```python
from build123d import *

# Parameters (mm, degrees)
SKETCH1_R                          = 76.2
MAIN_EXTRUDE_DEPTH                 = 50.5582
SKETCH4_R                          = 76.2
SKETCH4_R_2                        = 75.057
TURN_OUTSIDE_DEPTH                 = 37.846
SKETCH5_R                          = 74.295
EXTRUDE1_DEPTH                     = 0.9906
SKETCH7_R                          = 76.2
FACE_BOTTOM_DEPTH                  = 1.5367
SKETCH8_R                          = 76.2
SKETCH8_R_2                        = 75.057
TURN_REST_OF_OUTSIDE_DEPTH         = 12.1755
SKETCH3_R                          = 2.3876
PILOT_HOLE_FOR_BALL_DEPTH          = 12.446
SPHERICAL_BALL_ANGLE               = 180
CHAMFER1_SIZE                      = 16.002
F_5_16_0_3125_DIAMETER_HOLE1_D     = 7.9375
F_5_16_0_3125_DIAMETER_HOLE1_DEPTH = 0.508
RETAINER_HOLE_PATTERN_COUNT        = 3
M5X0_8_TAPPED_HOLE1_D              = 4.2
M5X0_8_TAPPED_HOLE1_DEPTH          = 66.675
M5X0_8_TAPPED_HOLE1_TIP            = 1.2618073


with BuildPart() as part:
    # Sketch1 → Main Extrude (new body)
    with BuildSketch(Plane(origin=(0, 0, 0), x_dir=(1, 0, 0), z_dir=(0, 1, 0))):
        with Locations(Location((0, 0, 0), (0, 0, 270))):  # turned: the seam where the file's is
            Circle(SKETCH1_R)
    extrude(amount=MAIN_EXTRUDE_DEPTH)

    # Sketch4 → Turn Outside (cut)
    with BuildSketch(Plane.XZ):
        with Locations(Location((0, 0, 0), (0, 0, 270))):  # turned: the seam where the file's is
            Circle(SKETCH4_R)
        with Locations(Location((0, 0, 0), (0, 0, 270))):  # turned: the seam where the file's is
            Circle(SKETCH4_R_2, mode=Mode.SUBTRACT)
    extrude(amount=-TURN_OUTSIDE_DEPTH, mode=Mode.SUBTRACT)

    # Sketch5 → Extrude1 (add)
    with BuildSketch(Plane.XZ):
        with Locations(Location((0, 0, 0), (0, 0, 90))):  # turned: the seam where the file's is
            Circle(SKETCH5_R)
    extrude(amount=EXTRUDE1_DEPTH)

    # Sketch7 → Face Bottom (cut)
    with BuildSketch(Plane(origin=(0, 50.5582, 0), x_dir=(-1, 0, 0), z_dir=(0, 1, 0))):
        with Locations(Location((0, 0, 0), (0, 0, 270))):  # turned: the seam where the file's is
            Circle(SKETCH7_R)
    extrude(amount=-FACE_BOTTOM_DEPTH, mode=Mode.SUBTRACT)

    # Sketch8 → Turn rest of outside (cut, through all)
    with BuildSketch(Plane.XZ.offset(-37.846)):
        Circle(SKETCH8_R)
        with Locations(Location((0, 0, 0), (0, 0, 270))):  # turned: the seam where the file's is
            Circle(SKETCH8_R_2, mode=Mode.SUBTRACT)
    extrude(amount=-TURN_REST_OF_OUTSIDE_DEPTH, mode=Mode.SUBTRACT)

    # Sketch3 → Pilot hole for ball (cut)
    with BuildSketch(Plane(origin=(0, 49.0215, 0), x_dir=(-1, 0, 0), z_dir=(0, 1, 0))):
        with Locations(Location((0, 0, 0), (0, 0, 90))):  # turned: the seam where the file's is
            Circle(SKETCH3_R)
    extrude(amount=-PILOT_HOLE_FOR_BALL_DEPTH, mode=Mode.SUBTRACT)

    # Sketch2 → Spherical Ball (revolve, cut)
    with BuildSketch(Plane(origin=(0, 49.5295, 0), x_dir=(-1, 0, 0), z_dir=(0, 1, 0))):
        with BuildLine():
            Line((12.499975, 0), (-12.499975, 0))
            ThreePointArc((-12.499975, 0), (0, -12.499975), (12.499975, 0))
        make_face()
    revolve(axis=Axis((-12.499975, 49.5295, 0), (-1, 0, 0)), revolution_arc=SPHERICAL_BALL_ANGLE, mode=Mode.SUBTRACT)

    # Chamfer1
    chamfer1_edges = [part.edges().sort_by_distance(p)[0] for p in [
        (0, 49.0215, 75.057),
    ]]
    chamfer(chamfer1_edges, length=CHAMFER1_SIZE)

    # 5_16 _0.3125_ Diameter Hole1
    with Locations(Plane(origin=(75.184, 0, 0), x_dir=(0, 0, -1), z_dir=(1, 0, 0))):
        with Locations((0, 7.5179)):
            Hole(F_5_16_0_3125_DIAMETER_HOLE1_D / 2, depth=F_5_16_0_3125_DIAMETER_HOLE1_DEPTH)

    # Sketch15 → M3x0.5 Retainer Hole (revolve, cut)
    with BuildSketch(Plane(origin=(-19.05, 49.0215, 0), x_dir=(0, 0, 1), z_dir=(1, 0, 0))):
        Polygon((0, 0), (0, 8.599675774), (1.25, 7.8486), (1.25, 0), align=None)
    m3x0_5_retainer_hole = revolve(axis=Axis((-19.05, 55.3715, 0), (0, -1, 0)), mode=Mode.SUBTRACT)

    # Retainer hole pattern: M3x0.5 Retainer Hole ×3 about axis
    retainer_hole_pattern_axis = Axis((0, 0, 0), (0, 1, 0))
    for i in range(1, RETAINER_HOLE_PATTERN_COUNT):
        add(m3x0_5_retainer_hole.rotate(retainer_hole_pattern_axis, i * 360 / RETAINER_HOLE_PATTERN_COUNT), mode=Mode.SUBTRACT)

    # M5x0.8 Tapped Hole1
    with Locations(Plane(origin=(74.676, 0, 0), x_dir=(0, 0, -1), z_dir=(1, 0, 0))):
        with Locations((0, 7.5179)):
            Hole(M5X0_8_TAPPED_HOLE1_D / 2, depth=M5X0_8_TAPPED_HOLE1_DEPTH)
            with Locations((0, 0, -(M5X0_8_TAPPED_HOLE1_DEPTH + M5X0_8_TAPPED_HOLE1_TIP / 2))):  # 118° drill point
                Cone(0, M5X0_8_TAPPED_HOLE1_D / 2, M5X0_8_TAPPED_HOLE1_TIP, mode=Mode.SUBTRACT)


solid = part.part
```
Geometry: final body of the model. Coordinates: model frame, mm. A direction names the side the tool comes from. Round coordinates to 2 decimals unless told otherwise and drop trailing zeros. Write each loop counter-clockwise with the first axis right and the second up, starting at its lowest first coordinate (ties: lowest second). Pieces come first, ordered by that corner, then holes. Notation, with made-up numbers: M 0.5,-15.5 L 33.5,-15.5 A37 cw 33.5,23.5 Z; hole C -9.5,48.5 d1. An arc over 180 degrees is marked long. Answer in a Markdown table with one row per item. Add a question column.
(1) Draft query along Y for faces 4 (the face through (74.676, 6, 2)), 5 (the face through (-73.663, -0.488, -9.672)), 6 (the face through (-58.409, 48.245, 12.97)), 7 (the face through (72.6, 0, -17)). Return one class per face: pulls with the +Y half, pulls with the -Y half, needs draft (parallel to the pull), parting line crosses it, or undercut.
(2) Cut plane A-A, the plane x = 0. Return the cut outline in (y, z) (1 decimal).
(3) Reachability of faces 1 (the face through (0, 36.576, 0)), 2 (the face through (74.864, 3.644, -0.86)), 3 (the face through (-14, 49.021, 1)) from +Z, -Z, +X, -X, +Y, -Y: full face, straight path, thin tool, end or side. Return the list, or none.
(4) Cut plane B-B, the plane y = 14. Return the cut outline in (x, z).
(5) Ray query, L1, parallel to X at y = 1, z = -10.5; L2, parallel to Z at x = 31, y = 7; L3, parallel to Y at x = 74, z = 0. Return the intervals inside material, ascending.
(6) Contact query for flat-ended pins moving along their axis: pin 1 (2.5 mm diameter, centred on y = 7.52, z = 0, fed in from +X); pin 2 (3 mm diameter, centred on x = -17.5, y = 32.5, fed in from +Z); pin 3 (4 mm diameter, centred on y = 6, z = -1, fed in from +X). Output: stop coordinate, or through.
Established:
| question | item | result |
|---|---|---|
| 1 | face 4 | undercut |
| 1 | face 5 | needs draft |
| 1 | face 6 | pulls with the +Y half |
| 1 | face 7 | pulls with the -Y half |
| 2 | outline | M -1,-74.3 L 0,-74.3 L 0,-75.1 L 33,-75.1 L 49,-59.1 L 49,-12.5 A12.5 cw 37.3,-2.4 L 36.6,-2.4 L 36.6,2.4 L 37.3,2.4 A12.5 cw 49,12.5 L 49,59.1 L 33,75.1 L 0,75.1 L 0,74.3 L -1,74.3 Z |
| 3 | face 1 | +Y |
| 3 | face 2 | +X |
| 3 | face 3 | +Z, -Z, +X, -X, +Y |
| 4 | outline | C 0,0 d150.11 |
| 5 | L1 | -74.32 to 74.32 |
| 5 | L2 | -68.36 to -2.04, 2.04 to 68.36 |
| 5 | L3 | -0.99 to 5.42, 9.62 to 34.08 |
| 6 | pin 1 | x = 7.49 |
| 6 | pin 2 | z = 73.33 |
| 6 | pin 3 | x = 74.68 |
